Geometry: final body of the model. Coordinates: model frame, mm. A direction names the side the tool comes from. Round coordinates to 2 decimals unless told otherwise and drop trailing zeros. Write each loop counter-clockwise with the first axis right and the second up, starting at its lowest first coordinate (ties: lowest second). Pieces come first, ordered by that corner, then holes. Notation, with made-up numbers: M 39.5,31.25 L 74.5,31.25 A19 cw 74.5,58.25 Z; hole C 85.5,-39 d9. An arc over 180 degrees is marked long. Answer as CSV lines item,"result". Start each with the question number.
Q1. Mould query, pull axis Z, two halves, no side actions, for faces 5 (the flat face through (-12.55, -3.32, -10.59)), 6 (the flat face through (12.668, -3.321, -8.039)), 7 (the flat face through (0, -4, 15.105)), 8 (the flat face through (12.525, -3.321, 10.573)). Classes: pulls with the +Z half, pulls with the -Z half, needs draft (parallel to the pull), parting line crosses it, or undercut.
Q2. Section query D-D on x = 4.14. Output: boundary loops of the cut face in (y, z) (3 decimals), and give its area (3 significant figures).
Q3. Ray query, probe 1 along Z at (x, y) = (-3.5, -4.2) (3 decimals); probe 2 along X at (y, z) = (-3.4, 14) (3 decimals); probe 3 along Y at (x, z) = (12.5, -2.5). Return the intervals inside material, ascending.
Q4. First-contact query: pin 1 (1.6 mm diameter, centred on x = -3, z = -19, fed in from -Y); pin 2 (1 mm diameter, centred on x = -0.5, y = -3.5, fed in from -Z); pin 3 (0.9 mm diameter, centred on y = -3, z = 7.5, fed in from +X). Flat tips, straight axial feed; report the tip coordinate or a pass-through.
Q5. Section query A-A on x = 0. Output: boundary loops of the cut face in (y, z) (3 decimals), and give its area (3 significant figures).
Q6. Section query B-B on z = 0. Output: boundary loops of the cut face in (x, y) (3 decimals).
Q7. Reachability of faces 1 (the flat face through (15.605, -2.95, -3.35)), 2 (the flat face through (15, -2.925, -10)), 3 (the flat face through (-15, -3.745, -10)), 4 (the cylindrical face through (7.969, -0.424, -16.246)) from +Z, -Z, +X, -X, +Y, -Y: full face, straight path, thin tool, end or side. Return the list, or none.
Q8. Section query C-C on x = 13. Output: boundary loops of the cut face in (y, z).
```python
from build123d import *

# Parameters (mm, degrees)
BOSS_EXTRUDE1_DEPTH     = 0.75
BOSS_EXTRUDE2_DEPTH     = 0.86
SKETCH3_R               = 17.905
BOSS_EXTRUDE3_DEPTH     = 1.5
SKETCH4_W               = 13.1
SKETCH4_H               = 19.04
BOSS_EXTRUDE4_DEPTH     = 0.8
SKETCH5_W               = 10.33
SKETCH5_H               = 13.26
BOSS_EXTRUDE5_DEPTH     = 1.96
SKETCH6_W               = 5.07
SKETCH6_H               = 2.08
BOSS_EXTRUDE6_DEPTH     = 1.91
SKETCH7_R               = 1.035
BOSS_EXTRUDE7_DEPTH     = 1.4
BOSS_EXTRUDE8_DEPTH     = 1.95
SKETCH9_W               = 1.91
SKETCH9_H               = 0.82
BOSS_EXTRUDE9_DEPTH     = 1.2
MIRROR2_COPY_1_SKETCH_W = 1.91
MIRROR2_COPY_1_SKETCH_H = 0.82
MIRROR2_COPY_1_DEPTH    = 1.2
SKETCH10_W              = 5.55
SKETCH10_H              = 7.5
BOSS_EXTRUDE10_DEPTH    = 2.65
CUT_EXTRUDE1_DEPTH      = 3.65
BOSS_EXTRUDE11_DEPTH    = 0.7
CUT_EXTRUDE2_DEPTH      = 10
CUT_EXTRUDE2_DEPTH_BACK = 10
FILLET1_R               = 0.5


with BuildPart() as part:
    # Sketch1 → Boss-Extrude1 (new body)
    with BuildSketch(Plane(origin=(0, 0, 0), x_dir=(1, 0, 0), z_dir=(0, 1, 0))):
        with BuildLine():
            Line((-6.25, 16.468932115), (6.25, 16.468932115))
            ThreePointArc((6.25, 16.468932115), (0, -17.615), (-6.25, 16.468932115))
        make_face()
    extrude(amount=BOSS_EXTRUDE1_DEPTH)

    # Sketch2 → Boss-Extrude2 (add)
    with BuildSketch(Plane(origin=(0, 0, 0), x_dir=(1, 0, 0), z_dir=(0, 1, 0))):
        with BuildLine():
            Line((6.59, 21.07), (-6.59, 21.07))
            Line((-6.59, 21.07), (-7.33, 17.670177364))
            ThreePointArc((-7.33, 17.670177364), (-7.956125045, 16.26379425), (-9.09, 15.222509649))
            ThreePointArc((-9.09, 15.222509649), (0, -17.73), (9.09, 15.222509649))
            ThreePointArc((9.09, 15.222509649), (7.956125045, 16.26379425), (7.33, 17.670177364))
            Line((7.33, 17.670177364), (6.59, 21.07))
        make_face()
    extrude(amount=-BOSS_EXTRUDE2_DEPTH)

    # Sketch3 → Boss-Extrude3 (add)
    with BuildSketch(Plane.XZ.offset(0.86)):
        with Locations(Location((0, 0, 0), (0, 0, 297.520154759))):
            Circle(SKETCH3_R)
    extrude(amount=BOSS_EXTRUDE3_DEPTH)

    # Sketch4 → Boss-Extrude4 (add)
    with BuildSketch(Plane.XZ.offset(2.36)):
        with Locations((0, 9.98)):
            Rectangle(SKETCH4_W, SKETCH4_H)
    extrude(amount=BOSS_EXTRUDE4_DEPTH)

    # Sketch5 → Boss-Extrude5 (add)
    with BuildSketch(Plane.XZ.offset(3.16)):
        with Locations((0, 8.475)):
            Rectangle(SKETCH5_W, SKETCH5_H)
    extrude(amount=BOSS_EXTRUDE5_DEPTH)

    # Sketch6 → Boss-Extrude6 (add)
    with BuildSketch(Plane.XZ.offset(3.16)):
        with Locations((-2.065, 18.16)):
            Rectangle(SKETCH6_W, SKETCH6_H)
    extrude(amount=BOSS_EXTRUDE6_DEPTH)

    # Sketch7 → Boss-Extrude7 (add)
    with BuildSketch(Plane.XZ.offset(3.16)):
        with Locations(Location((4.14, 17.95, 0), (0, 0, 270))):
            Circle(SKETCH7_R)
    extrude(amount=BOSS_EXTRUDE7_DEPTH)

    # Sketch8 → Boss-Extrude8 (add)
    with BuildSketch(Plane.XZ.offset(2.36)):
        Polygon((16, -7.445460012), (13.596778104, -11.25), (11.483144777, -9.914876724), (13.886366674, -6.110336737), align=None)
        Polygon((-16, -7.445460012), (-13.596778104, -11.25), (-11.483144777, -9.914876724), (-13.886366674, -6.110336737), align=None)
        Polygon((-16, 7.445460012), (-13.596778104, 11.25), (-11.483144777, 9.914876724), (-13.886366674, 6.110336737), align=None)
        Polygon((13.886366674, 6.110336737), (11.483144777, 9.914876724), (13.596778104, 11.25), (16, 7.445460012), align=None)
    extrude(amount=BOSS_EXTRUDE8_DEPTH)

    # Sketch9 → Boss-Extrude9 (add)
    with BuildSketch(Plane(origin=(-14.798389052, 0, -9.347730006), x_dir=(-0.5340493103180728, 0, 0.84545333055633), z_dir=(-0.8454533305563299, 0, -0.5340493103180727))):
        with Locations((0, -3.335)):
            Rectangle(SKETCH9_W, SKETCH9_H)
    boss_extrude9 = extrude(amount=BOSS_EXTRUDE9_DEPTH)

    # Mirror1: Boss-Extrude9 across plane
    add(boss_extrude9.mirror(Plane.XY))

    # Mirror2: Boss-Extrude9 across plane
    add(boss_extrude9.mirror(Plane(origin=(0, 0, 0), x_dir=(0, 0, 1), z_dir=(1, 0, 0))))

    # Mirror2 copy 1 sketch → Mirror2 copy 1 (add)
    with BuildSketch(Plane(origin=(14.798389052, 0, 9.347730006), x_dir=(0.5340493103180728, 0, -0.84545333055633), z_dir=(0.8454533305563299, 0, 0.5340493103180727))):
        with Locations((0, -3.335)):
            Rectangle(MIRROR2_COPY_1_SKETCH_W, MIRROR2_COPY_1_SKETCH_H)
    extrude(amount=MIRROR2_COPY_1_DEPTH)

    # Sketch10 → Boss-Extrude10 (add)
    with BuildSketch(Plane(origin=(0, -2.36, 0), x_dir=(-1, 0, 0), z_dir=(0, -1, 0))):
        with Locations((-16.48, 0)):
            Rectangle(SKETCH10_W, SKETCH10_H)
    extrude(amount=BOSS_EXTRUDE10_DEPTH)

    # Sketch11 → Cut-Extrude1 (cut)
    with BuildSketch(Plane(origin=(19.255, 0, 0), x_dir=(0, 0, -1), z_dir=(1, 0, 0))):
        Polygon((3.75, -5.01), (3.75, -3.91), (2.7, -2.36), (4.361270296, -2.36), (4.361270296, -9.207681493), (-4.361270296, -9.207681493), (-4.361270296, -2.36), (-2.7, -2.36), (-3.75, -3.91), (-3.75, -5.01), align=None)
    extrude(amount=-CUT_EXTRUDE1_DEPTH, mode=Mode.SUBTRACT)

    # Sketch12 → Boss-Extrude11 (add)
    with BuildSketch(Plane(origin=(0, 0, 0), x_dir=(1, 0, 0), z_dir=(0, 1, 0))):
        Polygon((-7.025339783, 16.718932115), (7.025339783, 16.718932115), (6.078293252, 21.07), (-6.078293252, 21.07), align=None)
    extrude(amount=BOSS_EXTRUDE11_DEPTH)

    # Sketch13 → Cut-Extrude2 (cut, two sides: drawn at the far end of the back side and taken through both)
    with BuildSketch(Plane(origin=(0, 0, 0), x_dir=(0, 0, -1), z_dir=(1, 0, 0)).offset(-CUT_EXTRUDE2_DEPTH_BACK)):
        with BuildLine():
            Line((16.718932115, 0.7), (20.225865386, 0.576368288))
            ThreePointArc((20.225865386, 0.576368288), (20.731401374, 0.410430291), (21.07, 0))
            Line((21.07, 0), (21.650216757, 1.081319804))
            Line((21.650216757, 1.081319804), (16.718932115, 1.620600457))
            Line((16.718932115, 1.620600457), (16.718932115, 0.7))
        make_face()
    extrude(amount=CUT_EXTRUDE2_DEPTH + CUT_EXTRUDE2_DEPTH_BACK, mode=Mode.SUBTRACT)

    # Fillet1
    fillet1_edges = [part.edges().sort_by_distance(p)[0] for p in [
        (6.152517901, 0.412074342, -20.728985619),
        (-6.152517901, 0.412074342, -20.728985619),
        (-6.643683018, 0.638184144, -18.47239875),
        (6.643683018, 0.638184144, -18.47239875),
    ]]
    fillet(fillet1_edges, radius=FILLET1_R)


solid = part.part
```
Entries:
1,face 5,"pulls with the -Z half"
1,face 6,"undercut"
1,face 7,"undercut"
1,face 8,"pulls with the +Z half"
2,outline,"M -5.12,1.845 L -3.16,1.845 L -3.16,0.46 L -2.36,0.46 L -2.36,-17.42 L -0.86,-17.42 L -0.86,-21.07 L 0,-21.07 A0.956 ccw 0.576,-20.226 L 0.7,-16.719 L 0,-16.719 L 0,-16.469 L 0.75,-16.469 L 0.75,17.122 L 0,17.122 L 0,17.24 L -0.86,17.24 L -0.86,17.42 L -2.36,17.42 L -2.36,19.5 L -3.16,19.5 L -3.16,18.985 L -4.56,18.985 L -4.56,16.915 L -3.16,16.915 L -3.16,15.105 L -5.12,15.105 Z"
2,area,"157 mm^2"
3,probe 1,"z = 1.845 to 15.105, 17.12 to 19.2"
3,probe 2,"x = -5.165 to 5.165"
3,probe 3,"y = -2.36 to 0.75"
4,pin 1,"stops at y = -0.86"
4,pin 2,"stops at z = 0.46"
4,pin 3,"stops at x = 16"
5,outline,"M -5.12,1.845 L -3.16,1.845 L -3.16,0.46 L -2.36,0.46 L -2.36,-17.905 L -0.86,-17.905 L -0.86,-21.07 L 0,-21.07 A0.956 ccw 0.576,-20.226 L 0.7,-16.719 L 0,-16.719 L 0,-16.469 L 0.75,-16.469 L 0.75,17.615 L 0,17.615 L 0,17.73 L -0.86,17.73 L -0.86,17.905 L -2.36,17.905 L -2.36,19.5 L -3.16,19.5 L -3.16,19.2 L -5.07,19.2 L -5.07,17.12 L -3.16,17.12 L -3.16,15.105 L -5.12,15.105 Z"
5,area,"160 mm^2"
6,outline,"M -17.905,-2.36 L 13.705,-2.36 L 13.705,-5.01 L 19.255,-5.01 L 19.255,-2.36 L 17.905,-2.36 L 17.905,-0.86 L 17.73,-0.86 L 17.73,0 L 17.615,0 L 17.615,0.75 L -17.615,0.75 L -17.615,0 L -17.73,0 L -17.73,-0.86 L -17.905,-0.86 Z"
7,face 1,"+X"
7,face 2,"-Z, +X"
7,face 3,"-Z, -X, -Y"
7,face 4,"-Z, +X, +Y"
8,outline,"M -4.31,-10.87 L -2.36,-10.87 L -2.36,-12.31 L -0.86,-12.31 L -0.86,-12.06 L 0,-12.06 L 0,-11.89 L 0.75,-11.89 L 0.75,11.89 L 0,11.89 L 0,12.06 L -0.86,12.06 L -0.86,12.31 L -2.36,12.31 L -2.36,10.87 L -4.31,10.87 L -4.31,7.51 L -2.36,7.51 L -2.36,-7.51 L -4.31,-7.51 Z"
